Build history of the part. All positions in model axes, mm. Face numbers are marked on the shaded views. A direction names the side the tool comes from. Round coordinates to 2 decimals unless told otherwise and drop trailing zeros. Write each loop counter-clockwise with the first axis right and the second up, starting at its lowest first coordinate (ties: lowest second). Pieces come first, ordered by that corner, then holes.
1) Saw through at B-B (z = 0). Write the cut outline in (x, y).
2) Wall check: probe 1 along X at (y, z) = (29, 0); probe 2 along Y at (x, z) = (3, -6.25); probe 3 along Z at (x, y) = (0.5, 33). Give the ranges that are in metal, low to high.
3) Saw through at A-A (x = 0). Write the cut outline in (y, z).
4) Saw through at C-C (y = 33). Write the cut outline in (x, z), plus the area to 3 significant figures.
5) Saw through at D-D (y = 55). Write the cut outline in (x, z).
6) Flat gauge pins, fed straight in: pin 1 (2 mm diameter, centred on x = -10, z = -0.5, fed in from +Y); pin 2 (2 mm diameter, centred on y = 32.5, z = -10.5, fed in from +X); pin 3 (6 mm diameter, centred on x = -5, z = -2.5, fed in from -Y). Where does each tip first touch, or does it go through?
7) Which spindle directions (+Z, -Z, +X, -X, +Y, -Y) get a long thin tool onto all of the face, cutting with end or side? Do the marked faces 1, 2 and 3. Say none if no direction does.
from build123d import *

# Parameters (mm, degrees)
ENL_V_MAT_EXTRU_1_DEPTH                   = 15
TROU_TARAUD_M31_D                         = 2.5
TROU_TARAUD_M31_DEPTH                     = 8.5
TROU_TARAUD_M31_TIP                       = 0.751075774
ESQUISSE5_W                               = 0.7
ESQUISSE5_H                               = 3.8
BOSS_EXTRU_1_DEPTH                        = 6.7
CHANFREIN1_SIZE                           = 1
ESQUISSE6_R                               = 0.8
ENL_V_MAT_EXTRU_2_DEPTH                   = 6.7
R_P_TITION_CIRCULAIRE1_COUNT              = 2
CHANFREIN1_OF_R_P_TITION_CIRCULAIRE1_SIZE = 1
ENL_V_MAT_EXTRU_4_DEPTH                   = 90.145947749
ENL_V_MAT_EXTRU_4_DEPTH_BACK              = 90.145947749
ESQUISSE7_R                               = 19
ESQUISSE7_R_2                             = 1.6


with BuildPart() as part:
    # Esquisse1 → Révolution1 (revolve)
    with BuildSketch(Plane.XY, mode=Mode.PRIVATE) as r_volution1_sk:
        with BuildLine():
            Line((0, 0), (-1.6, 0))
            Line((-1.6, 0), (-1.6, 2.6))
            Line((-1.6, 2.6), (-5.075, 2.6))
            Line((-5.075, 2.6), (-5.075, 4.5))
            Line((-5.075, 4.5), (-19, 4.5))
            Line((-19, 4.5), (-19, 58))
            Line((-19, 58), (-17.85, 58))
            Line((-17.85, 58), (-17.85, 60))
            ThreePointArc((-17.85, 60), (-17.410660172, 61.060660172), (-16.35, 61.5))
            Line((-16.35, 61.5), (-6.5, 61.5))
            Line((-6.5, 61.5), (-6.5, 65.8))
            Line((-6.5, 65.8), (-1.6, 65.8))
            Line((-1.6, 65.8), (-1.6, 85))
            Line((-1.6, 85), (0, 85))
            Line((0, 85), (0, 0))
        make_face()
    revolve(r_volution1_sk.sketch.rotate(Axis((0, 0, 0), (0, 1, 0)), 270), axis=Axis((0, 0, 0), (0, 1, 0)))

    # Esquisse2 → Enlèv. mat.-Extru.1 (cut)
    with BuildSketch(Plane(origin=(0, 85, 0), x_dir=(1, 0, 0), z_dir=(0, 1, 0))):
        with BuildLine():
            Line((-1.161895004, -1.1), (1.161895004, -1.1))
            ThreePointArc((1.161895004, -1.1), (0, -1.6), (-1.161895004, -1.1))
        make_face()
    extrude(amount=-ENL_V_MAT_EXTRU_1_DEPTH, mode=Mode.SUBTRACT)

    # Trou taraudé M31
    with Locations(Plane(origin=(0, 61.5, 0), x_dir=(-1, 0, 0), z_dir=(0, 1, 0))):
        with Locations((12.5, 0), (-12.5, 0)):
            Hole(TROU_TARAUD_M31_D / 2, depth=TROU_TARAUD_M31_DEPTH)
            with Locations((0, 0, -(TROU_TARAUD_M31_DEPTH + TROU_TARAUD_M31_TIP / 2))):  # 118° drill point
                Cone(0, TROU_TARAUD_M31_D / 2, TROU_TARAUD_M31_TIP, mode=Mode.SUBTRACT)

    # Esquisse5 → Boss.-Extru.1 (add)
    with BuildSketch(Plane.XZ.offset(-4.5)):
        with Locations((-13.95, 0)):
            Rectangle(ESQUISSE5_W, ESQUISSE5_H)
    boss_extru_1 = extrude(amount=BOSS_EXTRU_1_DEPTH)

    # Chanfrein1
    chanfrein1_edges = [part.edges().sort_by_distance(p)[0] for p in [
        (-13.95, -2.2, -1.9),
        (-13.95, -2.2, 1.9),
    ]]
    chamfer(chanfrein1_edges, length=CHANFREIN1_SIZE)

    # Esquisse6 → Enlèv. mat.-Extru.2 (cut)
    with BuildSketch(Plane.ZY.offset(14.3)):
        Circle(ESQUISSE6_R)
    enl_v_mat_extru_2 = extrude(amount=-ENL_V_MAT_EXTRU_2_DEPTH, mode=Mode.SUBTRACT)

    # Répétition circulaire1: Boss.-Extru.1, Enlèv. mat.-Extru.2 ×2 about axis
    r_p_tition_circulaire1_axis = Axis((0, 0, 0), (0, 1, 0))
    add([boss_extru_1.rotate(r_p_tition_circulaire1_axis, i * 360 / R_P_TITION_CIRCULAIRE1_COUNT) for i in range(1, R_P_TITION_CIRCULAIRE1_COUNT)])
    add([enl_v_mat_extru_2.rotate(r_p_tition_circulaire1_axis, i * 360 / R_P_TITION_CIRCULAIRE1_COUNT) for i in range(1, R_P_TITION_CIRCULAIRE1_COUNT)], mode=Mode.SUBTRACT)

    # Chanfrein1 of Répétition circulaire1
    chanfrein1_of_r_p_tition_circulaire1_edges = [part.edges().sort_by_distance(p)[0] for p in [
        (13.95, -2.2, 1.9),
        (13.95, -2.2, -1.9),
    ]]
    chamfer(chanfrein1_of_r_p_tition_circulaire1_edges, length=CHANFREIN1_OF_R_P_TITION_CIRCULAIRE1_SIZE)

    # Esquisse7 → Enlèv. mat.-Extru.4 (cut, two sides: drawn at the far end of the back side and taken through both)
    with BuildSketch(Plane.XZ.offset(-ENL_V_MAT_EXTRU_4_DEPTH_BACK)):
        Circle(ESQUISSE7_R)
        with Locations(Location((0, 0, 0), (0, 0, 270))):
            Circle(ESQUISSE7_R_2, mode=Mode.SUBTRACT)
    extrude(amount=ENL_V_MAT_EXTRU_4_DEPTH + ENL_V_MAT_EXTRU_4_DEPTH_BACK, mode=Mode.SUBTRACT)

    # Esquisse9 → Révolution2 (revolve)
    with BuildSketch(Plane.XY, mode=Mode.PRIVATE) as r_volution2_sk:
        with BuildLine():
            Line((0, 15), (11.5, 15))
            ThreePointArc((11.5, 15), (12.914213562, 15.585786438), (13.5, 17))
            Line((13.5, 17), (13.5, 43))
            ThreePointArc((13.5, 43), (12.914213562, 44.414213562), (11.5, 45))
            Line((11.5, 45), (0, 45))
            Line((0, 45), (0, 44.5))
            Line((0, 44.5), (10, 44.5))
            Line((10, 44.5), (10, 15.5))
            Line((10, 15.5), (0, 15.5))
            Line((0, 15.5), (0, 15))
        make_face()
    revolve(r_volution2_sk.sketch.rotate(Axis((0, 0, 0), (0, 1, 0)), 90), axis=Axis((0, 0, 0), (0, 1, 0)))


solid = part.part
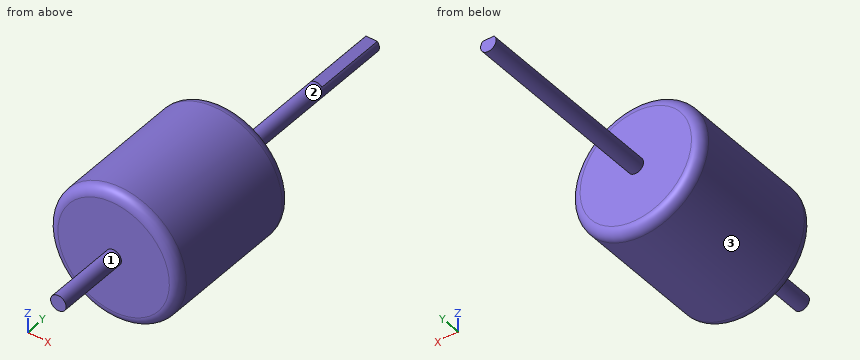
Evaluation:
1. outline: (-13.5, 17) arc R2 ccw to (-11.5, 15) - (-1.6, 15) - (-1.6, 0) - (1.6, 0) - (1.6, 15) - (11.5, 15) arc R2 ccw to (13.5, 17) - (13.5, 43) arc R2 ccw to (11.5, 45) - (1.6, 45) - (1.6, 85) - (-1.6, 85) - (-1.6, 45) - (-11.5, 45) arc R2 ccw to (-13.5, 43) - close; hole (-10, 15.5) - (-1.6, 15.5) - (-1.6, 44.5) - (-10, 44.5) - close; hole (1.6, 15.5) - (10, 15.5) - (10, 44.5) - (1.6, 44.5) - close
2. probe 1: x = -13.5 to -10, -1.6 to 1.6, 10 to 13.5
2. probe 2: y = 15 to 15.5, 44.5 to 45
2. probe 3: z = -13.49 to -9.99, -1.52 to 1.52, 9.99 to 13.49
3. outline: (0, -1.6) - (15, -1.6) - (15, -11.5) arc R2 ccw to (17, -13.5) - (43, -13.5) arc R2 ccw to (45, -11.5) - (45, -1.6) - (85, -1.6) - (85, 1.1) - (70, 1.1) - (70, 1.6) - (45, 1.6) - (45, 11.5) arc R2 ccw to (43, 13.5) - (17, 13.5) arc R2 ccw to (15, 11.5) - (15, 1.6) - (0, 1.6) - close; hole (15.5, -10) - (44.5, -10) - (44.5, -1.6) - (15.5, -1.6) - close; hole (15.5, 1.6) - (44.5, 1.6) - (44.5, 10) - (15.5, 10) - close
4. outline: circle Ø27 at (0, 0); circle Ø3.2 at (0, 0); hole circle Ø20 at (0, 0)
4. area: 266 mm2
5. outline: circle Ø3.2 at (0, 0)
6. pin 1: stops at y = 45
6. pin 2: stops at x = 9.59
6. pin 3: stops at y = 15
7. face 1: -Y
7. face 2: +Y
7. face 3: +Y, -Y
